Geometry check sheet. Reference: the model listing, model coordinates, mm. A direction names the side the tool comes from. Round coordinates to 2 decimals unless told otherwise and drop trailing zeros. Loops run counter-clockwise (first coordinate to the right, second up) from the corner with the lowest first, then second, coordinate; pieces in that order, holes last. Notation, with made-up numbers: (78.5, -27) - (116.5, -27) arc R27 cw to (116.5, -11) - close; hole circle Ø11 at (-12.5, -26). An arc over 180 degrees is marked (long way). Answer as CSV lines item,"result". Start each with the question number.
1) Access from +Z, -Z, +X, -X, +Y, -Y to the whole of each face (thin tool, end or side, straight path). Record for faces 1 (the flat face through (0, -27.5, 6)), 2 (the flat face through (-22, 0, -3)), 3 (the flat face through (30, 0, 9)).
2) Cross-section at B-B on z = 5.5. Record the boundary of the cut face in (x, y).
3) Thickness scan on line 1 along X through (y, z) = (16, 3); line 2 along Y through (x, z) = (12, 13.5). Record the ranges inside material, lowest first.
4) Draft check along Y on faces 4 (the cylindrical face through (0.42, -27.594, -2.719)), 5 (the flat face through (0, 28.5, 14)), 6 (the cylindrical face through (27.594, -0.42, -2.719)). Enter one of: released by +Y, released by -Y, zero draft, split by the parting line, or undercut.
5) Cross-section at D-D on z = -2. Record the boundary of the cut face in (x, y) (3 decimals).
6) Cross-section at A-A on y = 0.5. Record the boundary of the cut face in (x, z), and give its area (3 significant figures).
7) Depth check by flat-ended pin: P1, Ø12, axis at x = -20.5, y = -7, coming from the -Z side; P2, Ø2.5, axis at x = 8.5, z = -3.5, coming from the -Y side; P3, Ø1, axis at x = 8.5, z = -2, coming from the +Y side; P4, Ø5.5, axis at y = -6, z = -3.5, coming from the -X side. Enter the tip coordinate at first touch or a pass-through.
from build123d import *

# Parameters (mm, degrees)
F0_W     = 60
F0_H     = 60
F0_W_2   = 55
F0_H_2   = 55
F1_DEPTH = 15
F2_W     = 60
F2_H     = 60
F2_W_2   = 55
F2_H_2   = 55
F3_DEPTH = 5
F4_W     = 57
F4_H     = 57
F4_W_2   = 55
F4_H_2   = 55
F5_DEPTH = 3
F6_R     = 8
F7_W     = 44
F7_H     = 44
F8_DEPTH = 5


with BuildPart() as f1:
    # F0 (on Top) → F1 (new body)
    with BuildSketch(Plane.XY):
        Rectangle(F0_W, F0_H)
        Rectangle(F0_W_2, F0_H_2, mode=Mode.SUBTRACT)
    extrude(amount=F1_DEPTH)

    # F2 (on face) → F3 (join)
    with BuildSketch(Plane(origin=(0, 0, 0), x_dir=(1, 0, 0), z_dir=(0, 0, -1))):
        Rectangle(F2_W, F2_H)
        Rectangle(F2_W_2, F2_H_2, mode=Mode.SUBTRACT)
        Rectangle(F2_W_2, F2_H_2)
    extrude(amount=F3_DEPTH)

    # F4 (on face) → F5 (cut)
    with BuildSketch(Plane.XY.offset(15)):
        Rectangle(F4_W, F4_H)
        Rectangle(F4_W_2, F4_H_2, mode=Mode.SUBTRACT)
    extrude(amount=-F5_DEPTH, mode=Mode.SUBTRACT)

    # F6
    f6_edges = [f1.edges().sort_by_distance(p)[0] for p in [
        (-30, 0, -5),
        (30, 0, -5),
        (0, 30, -5),
        (0, -30, -5),
    ]]
    fillet(f6_edges, radius=F6_R)

    # F7 (on face) → F8 (cut)
    with BuildSketch(Plane(origin=(0, 0, -5), x_dir=(1, 0, 0), z_dir=(0, 0, -1))):
        Rectangle(F7_W, F7_H)
    extrude(amount=-F8_DEPTH, mode=Mode.SUBTRACT)


solid = f1.part
Answer block:
1,face 1,"+Z"
1,face 2,"+Z, -Z"
1,face 3,"+Z, -Z, +X, +Y, -Y"
2,outline,"(-30, -30) - (30, -30) - (30, 30) - (-30, 30) - close; hole (-27.5, -27.5) - (27.5, -27.5) - (27.5, 27.5) - (-27.5, 27.5) - close"
3,line 1,"x = -30 to -27.5, 27.5 to 30"
3,line 2,"y = -30 to -28.5, 28.5 to 30"
4,face 4,"released by -Y"
4,face 5,"undercut"
4,face 6,"zero draft"
5,outline,"(-28.245, -28.245) - (28.245, -28.245) - (28.245, 28.245) - (-28.245, 28.245) - close; hole (-22, -22) - (22, -22) - (22, 22) - (-22, 22) - close"
6,outline,"(-30, 3) arc R8 ccw to (-22, -5) - (-22, 0) - (-27.5, 0) - (-27.5, 12) - (-28.5, 12) - (-28.5, 15) - (-30, 15) - close; (22, -5) arc R8 ccw to (30, 3) - (30, 15) - (28.5, 15) - (28.5, 12) - (27.5, 12) - (27.5, 0) - (22, 0) - close"
6,area,"122 mm^2"
7,P1,"stops at z = -5"
7,P2,"stops at y = -28.04"
7,P3,"stops at y = 28.61"
7,P4,"stops at x = -29.07"
